```python
from build123d import *
from build123d.topology import SkipClean

# Parameters (mm, degrees)
SKETCH_1_R               = 4
EXTRUDE_1_DEPTH          = 40
CUT_EXTRUDE_1_DEPTH      = 53.194647057
CUT_EXTRUDE_1_DEPTH_BACK = 53.194647057


with BuildPart() as part:
    # Sketch 1 → Extrude 1 (new, symmetric)
    with BuildSketch(Plane.XY):
        Circle(SKETCH_1_R)
    extrude(amount=EXTRUDE_1_DEPTH, both=True)

    # Sketch 2 → Revolve 2 (revolve)
    with SkipClean():  # the faces are left unmerged after this step: merging them gives an invalid solid
        with BuildSketch(Plane(origin=(0, 0, 0), x_dir=(1, 0, 0), z_dir=(0, 1, 0)), mode=Mode.PRIVATE) as revolve_2_sk:
            with BuildLine():
                ThreePointArc((6.403124237, 45), (4.527692569, 49.527692569), (0, 51.403124237))
                Line((0, 51.403124237), (0, 48.5))
                ThreePointArc((0, 48.5), (2.474873734, 47.474873734), (3.5, 45))
                ThreePointArc((3.5, 45), (2.474873734, 42.525126266), (0, 41.5))
                Line((0, 41.5), (0, 38.596875763))
                ThreePointArc((0, 38.596875763), (4.527692569, 40.472307431), (6.403124237, 45))
            make_face()
            with BuildLine():
                Line((0, 48.5), (0, 51.403124237))
                ThreePointArc((0, 51.403124237), (-6.403124237, 45), (0, 38.596875763))
                Line((0, 38.596875763), (0, 41.5))
                ThreePointArc((0, 41.5), (-3.5, 45), (0, 48.5))
            make_face()
            with BuildLine():
                ThreePointArc((0, -38.596875763), (-6.403124237, -45), (0, -51.403124237))
                Line((0, -51.403124237), (0, -48.5))
                ThreePointArc((0, -48.5), (-3.5, -45), (0, -41.5))
                Line((0, -41.5), (0, -38.596875763))
            make_face()
            with BuildLine():
                Line((0, -48.5), (0, -51.403124237))
                ThreePointArc((0, -51.403124237), (4.527692569, -49.527692569), (6.403124237, -45))
                ThreePointArc((6.403124237, -45), (4.527692569, -40.472307431), (0, -38.596875763))
                Line((0, -38.596875763), (0, -41.5))
                ThreePointArc((0, -41.5), (2.474873734, -42.525126266), (3.5, -45))
                ThreePointArc((3.5, -45), (2.474873734, -47.474873734), (0, -48.5))
            make_face()
        revolve(revolve_2_sk.sketch.rotate(Axis((0, 0, -51.403124237), (0, 0, 1)), 180), axis=Axis((0, 0, -51.403124237), (0, 0, 1)))

    # Sketch 3 → Cut-Extrude 1 (cut, two sides: drawn at the far end of the back side and taken through both)
    with SkipClean():  # the faces are left unmerged after this step: merging them gives an invalid solid
        with BuildSketch(Plane(origin=(0, 0, 0), x_dir=(0, 0, -1), z_dir=(1, 0, 0)).offset(-CUT_EXTRUDE_1_DEPTH_BACK)):
            Polygon((-33, 4), (-40, 1.5), (-53, 1.5), (-53, 8), (-33, 8), align=None)
            Polygon((-33, -8), (-33, -4), (-40, -1.5), (-53, -1.5), (-53, -8), align=None)
            Polygon((33, -4), (40, -1.5), (53, -1.5), (53, -8), (33, -8), align=None)
            Polygon((33, 8), (33, 4), (40, 1.5), (53, 1.5), (53, 8), align=None)
        extrude(amount=CUT_EXTRUDE_1_DEPTH + CUT_EXTRUDE_1_DEPTH_BACK, mode=Mode.SUBTRACT)


solid = part.part
```
The model under review builds one solid part; all positions refer to its coordinate system, in mm. A direction names the side the tool comes from. Round coordinates to 2 decimals unless told otherwise and drop trailing zeros. Write each loop counter-clockwise with the first axis right and the second up, starting at its lowest first coordinate (ties: lowest second). Pieces come first, ordered by that corner, then holes. Notation, with made-up numbers: (63, 79) - (82, 79) arc R16 cw to (82, 85) - close; hole circle Ø4 at (50.5, -9.5). An arc over 180 degrees is marked (long way). One line per question, with ' | ' between items.
Item 1: Add section A-A, the plane z = 0. Give the boundary of the cut face in (x, y).
Resolved:
outline: circle Ø8 at (0, 0)
Item 2: For faces 4 (the face through (-1.5, 1.5, 48)), 5 (the face through (-1.5, -1.5, 48)), 6 (the face through (-1.5, -1.5, -48)), 7 (the face through (-0.1, 2.5, -37.2)), list the 3-axis set-ups (+Z, -Z, +X, -X, +Y, -Y) from which the entire face can be reached by the end or side of a thin tool; tool diameter is ignored.
Resolved:
face 4: +Z, +X, -X, +Y | face 5: +Z, +X, -X, -Y | face 6: -Z, +X, -X, -Y | face 7: -Z, +X, -X, +Y
Item 3: Add section B-B, the plane y = 3. Give the boundary of the cut face in (x, z).
Resolved:
outline: (-2.65, -35.8) - (2.65, -35.8) - (2.65, 35.8) - (-2.65, 35.8) - close
Item 4: For P1, Ø1.5, axis at y = 1, z = 9, coming from the -X side; P2, Ø3.5, axis at x = 1.5, z = -46.5, coming from the +Y side; P3, Ø1, axis at x = -3.5, z = 18, coming from the -Y side, all flat-tipped, find the tip position at first contact; note any pin that passes through.
Resolved:
P1: stops at x = -3.99 | P2: stops at y = 1.5 | P3: stops at y = -2.65
Item 5: The part is to be moulded in two halves that separate along Y. For faces 1 (the face through (-1.5, 1.5, -48)), 2 (the face through (-0.1, -2.5, 37.2)), 3 (the face through (-4, 0, 1)), say which applies: pulls with the +Y half, pulls with the -Y half, needs draft (parallel to the pull), parting line crosses it, or undercut.
Resolved:
face 1: pulls with the +Y half | face 2: pulls with the -Y half | face 3: parting line crosses it
